Part model, mm, in its own coordinate system. Face numbers are marked on the shaded views. A direction names the side the tool comes from. Coordinates: 2 decimals unless noted, no trailing zeros. Loops run counter-clockwise (first coordinate to the right, second up) from the corner with the lowest first, then second, coordinate; pieces in that order, holes last. Notation, with made-up numbers: (-7.75, -13.75) - (6.25, -13.75) arc R26 ccw to (6.25, 14.25) - close; hole circle Ø2 at (-20.75, 84). An arc over 180 degrees is marked (long way). One line per question, with ' | ' between items. Start each with the question number.
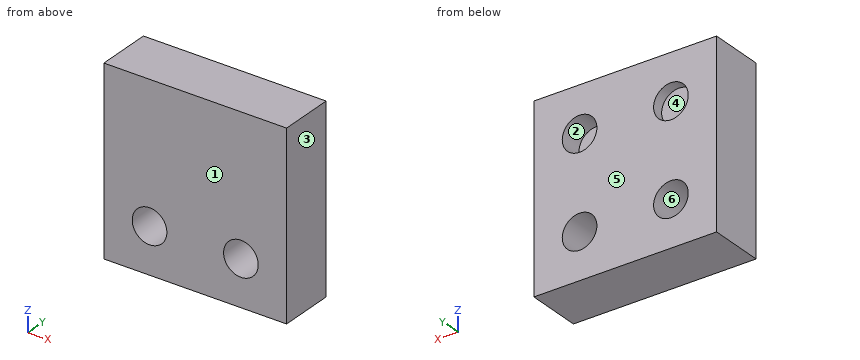
Autodesk Inventor part; units mm, degrees
ref_plane "YZ Plane" through (0, 0, 0) normal (1, 0, 0) x (0, 1, 0)
ref_plane "XY Plane" through (0, 0, 0) normal (0, 0, 1) x (1, 0, 0)
sketch "Sketch1" plane through (0, 0, 0) normal (0, 1, 0) x (-1, 0, 0)
  line L0 (15, 15) -> (0, 15)
  line L1 (0, 15) -> (0, 0)
  line L2 (0, 0) -> (15, 0)
  line L3 (15, 0) -> (15, 15)
  dimension "d0" = 15
  dimension "d1" = 15
extrude "Extrusion1" add sketch "Sketch1" along normal blind 13
sketch "Sketch2" plane through (0, 13, 0) normal (0, 1, 0) x (1, 0, 0)
  line L0 (-15, -15) -> (0, -15) construction
  line L1 (0, -15) -> (0, 0) construction
  line L2 (0, 0) -> (-15, 0) construction
  line L3 (-15, 0) -> (-15, -15) construction
  line L4 (-15, 0) -> (-15, -15) construction
  line L5 (-15, -7.5) -> (0, -7.5) construction
  line L6 (-15, -7.5) -> (0, -7.5)
  line L7 (0, -7.5) -> (0, 0)
  line L8 (0, 0) -> (-15, 0)
  line L9 (-15, 0) -> (-15, -7.5)
extrude "Extrusion2" cut sketch "Sketch2" against normal blind 4.1
sketch "Sketch3" plane through (0, 13, 0) normal (0, 1, 0) x (1, 0, 0)
  line L0 (0, -7.5) -> (-15, -7.5) construction
  line L1 (-15, -7.5) -> (-15, -15) construction
  line L2 (-15, -15) -> (0, -15) construction
  line L3 (0, -15) -> (0, -7.5) construction
  line L4 (-15, -15) -> (0, -15) construction
  line L5 (-7.5, -15) -> (-7.5, -7.5) construction
  line L6 (-15, -15) -> (-7.5, -15)
  line L7 (-7.5, -15) -> (-7.5, -7.5)
  line L8 (-7.5, -7.5) -> (-15, -7.5)
  line L9 (-15, -7.5) -> (-15, -15)
  point P0 (0, 0)
extrude "Extrusion3" add sketch "Sketch3" along normal blind 1
sketch "Sketch4" plane through (0, 8.9, 0) normal (0, 1, 0) x (1, 0, 0)
  line L0 (0, 0) -> (0, -7.5) construction
  line L1 (-15, 0) -> (0, 0) construction
  line L2 (-15, -7.5) -> (-15, 0) construction
  line L3 (0, -7.5) -> (-15, -7.5) construction
  line L4 (-7.5, -7.5) -> (-7.5, 0) construction
  line L5 (-7.5, -7.5) -> (0, -7.5)
  line L6 (0, -7.5) -> (0, 0)
  line L7 (0, 0) -> (-7.5, 0)
  line L8 (-7.5, 0) -> (-7.5, -7.5)
extrude "Extrusion4" add sketch "Sketch4" along normal blind 1
sketch "Sketch5" plane through (0, 14, 0) normal (0, 1, 0) x (1, 0, 0)
  line L0 (-15, -15) -> (-7.5, -15) construction
  line L1 (-7.5, -15) -> (-7.5, -7.5) construction
  line L2 (-7.5, -7.5) -> (-15, -7.5) construction
  line L3 (-15, -7.5) -> (-15, -15) construction
  point P0 (0, 0)
  point P1 (-11.25, -11.25)
  point P2 (-11.25, -11.25)
sketch "Sketch6" plane through (0, 13, 0) normal (0, 1, 0) x (1, 0, 0)
  line L0 (-7.5, -7.5) -> (-7.5, -15) construction
  line L1 (-7.5, -15) -> (0, -15) construction
  line L2 (0, -15) -> (0, -7.5) construction
  line L3 (0, -7.5) -> (-7.5, -7.5) construction
  point P0 (0, 0)
  point P1 (-3.75, -11.25)
sketch "Sketch7" plane through (0, 9.9, 0) normal (0, 1, 0) x (1, 0, 0)
  line L0 (0, -7.5) -> (0, 0) construction
  line L1 (0, 0) -> (-7.5, 0) construction
  line L2 (-7.5, 0) -> (-7.5, -7.5) construction
  line L3 (0, -7.5) -> (-7.5, -7.5) construction
  point P0 (-3.75, -3.75)
sketch "Sketch8" plane through (0, 8.9, 0) normal (0, 1, 0) x (1, 0, 0)
  line L0 (-7.5, -7.5) -> (-7.5, 0) construction
  line L1 (-15, 0) -> (-7.5, 0) construction
  line L2 (-15, -7.5) -> (-15, 0) construction
  line L3 (-7.5, -7.5) -> (-15, -7.5) construction
  point P0 (0, 0)
  point P1 (-11.25, -3.75)
hole "Hole1" at (-11.25, 14, 11.25) direction (0, -1, 0) diameter 2.8448 depth 10.414 counterbore diameter 5.37 counterbore depth 2.85
hole "Hole2" at (-3.75, 13, 11.25) direction (0, -1, 0) diameter 2.8448 depth 10.414 counterbore diameter 5.37 counterbore depth 2.85
hole "Hole3" at (-11.25, 8.9, 3.75) direction (0, -1, 0) diameter 2.8448 depth 10.414 counterbore diameter 5.37 counterbore depth 2.85
hole "Hole4" at (-3.75, 9.9, 3.75) direction (0, -1, 0) diameter 2.8448 depth 10.414 counterbore diameter 5.37 counterbore depth 2.85
ref_plane "Work Plane1" through (0, 4.5, 0) normal (0, 1, 0) x (-1, 0, 0)
split "Split1" plane through (0, 4.5, 0) removes the side toward (0, 1, 0)
properties part number "screwprint"
1) Band-saw the part on B-B on z = 3.75. List the corners of the cut face in (x, y), then the cut area to 3 significant figures.
2) Tool access for the marked faces 1 and 2: list every direction of +Z, -Z, +X, -X, +Y, -Y with a clear straight run to the whole face (end or side of a thin tool).
3) Mould opens along X. For the marked faces 3, 4, 5 and 6 say: +X half, -X half, draft (parallel to the pull), parting line (faces both ways), or undercut.
4) Band-saw the part on C-C on y = 3. List the corners of the cut face in (x, z), then the cut area to 3 significant figures.
5) Wall check: line 1 along X through (y, z) = (1.05, 3.75); line 2 along Z through (x, y) = (-11.25, 3.85); line 3 along Z through (x, y) = (-11.25, 1.25). Give the ranges that are in metal, low to high. Write a range as [from, to].
6) Band-saw the part on D-D on y = 1.95. List the corners of the cut face in (x, z), then the cut area to 3 significant figures.
7) Pin check, flat tips, straight feed: pin 1 Ø3 at (x, z) = (-4, 11) entering from +Y; pin 2 Ø2.5 at (x, z) = (-11.25, 11.25) entering from +Y. Stop position of each tip, or through.
8) Band-saw the part on A-A on x = -11.25. List the corners of the cut face in (y, z), then the cut area to 3 significant figures.
Values found:
1) outline: (-15, 0) - (-12.67, 0) - (-12.67, 4.5) - (-15, 4.5) - close; (-9.83, 0) - (-5.17, 0) - (-5.17, 4.5) - (-9.83, 4.5) - close; (-2.33, 0) - (0, 0) - (0, 4.5) - (-2.33, 4.5) - close | area: 41.9 mm²
2) face 1: +Z, -Z, +X, -X, -Y | face 2: +Y
3) face 3: +X half | face 4: undercut | face 5: draft | face 6: undercut
4) outline: (-15, 0) - (0, 0) - (0, 15) - (-15, 15) - close; hole circle Ø2.84 at (-11.25, 3.75); hole circle Ø2.84 at (-3.75, 3.75); hole circle Ø2.84 at (-3.75, 11.25) | area: 206 mm²
5) line 1: [-15, -12.67], [-9.83, -5.17], [-2.33, 0] | line 2: [0, 2.33], [5.17, 9.83], [12.67, 15] | line 3: [0, 2.33], [5.17, 15]
6) outline: (-15, 0) - (0, 0) - (0, 15) - (-15, 15) - close; hole circle Ø2.84 at (-11.25, 3.75); hole circle Ø2.84 at (-3.75, 3.75) | area: 212 mm²
7) pin 1: y = 4.5 | pin 2: y = 3.59
8) outline: (0, 0) - (4.5, 0) - (4.5, 2.33) - (0, 2.33) - close; (0, 5.17) - (4.5, 5.17) - (4.5, 9.83) - (3.59, 9.83) - (3.59, 12.67) - (4.5, 12.67) - (4.5, 15) - (0, 15) - close | area: 52.1 mm²
